Geometry: final body of the model. Coordinates: model frame, mm. A direction names the side the tool comes from. Coordinates: 2 decimals unless noted, no trailing zeros. Write each loop counter-clockwise with the first axis right and the second up, starting at its lowest first coordinate (ties: lowest second). Pieces come first, ordered by that corner, then holes. Notation, with made-up numbers: (-34, -2) - (-27, -2) arc R28 cw to (-27, 34) - close; hole circle Ø2 at (47, 83). An arc over 180 degrees is marked (long way). Put each result on its own line as item: value.
```python
from build123d import *

# Parameters (mm, degrees)
EXTRUDE_1_DEPTH    = 3
CHAMFER1_SIZE      = 110
SKETCH1_R          = 2.5
CUT_EXTRUDE1_DEPTH = 10
SKETCH2_R          = 1.6
CUT_EXTRUDE2_DEPTH = 10
CUT_EXTRUDE3_DEPTH = 10
SKETCH4_R          = 1.6
CUT_EXTRUDE4_DEPTH = 8
SKETCH5_R          = 1.5
CUT_EXTRUDE5_DEPTH = 3
SKETCH6_R          = 1.6
CUT_EXTRUDE6_DEPTH = 3
CHAMFER2_SIZE      = 10
SKETCH7_R          = 1.6
CUT_EXTRUDE7_DEPTH = 10


with BuildPart() as part:
    # 草图1 → 凸台-拉伸1 (new body)
    with BuildSketch(Plane.XY):
        Polygon((-225, 205), (-228, 205), (-228, 175), (-225, 175), (-225, 50), (-228, 50), (-228, 20), (-225, 20), (-225, -105), (-228, -105), (-228, -135), (-225, -135), (-225, -285), (225, -285), (225, -135), (228, -135), (228, -105), (225, -105), (225, 20), (228, 20), (228, 50), (225, 50), (225, 175), (228, 175), (228, 205), (225, 205), (225, 285), (-225, 285), align=None)
    extrude(amount=EXTRUDE_1_DEPTH)

    # Chamfer1
    chamfer1_edges = [part.edges().sort_by_distance(p)[0] for p in [
        (225, -285, 1.5),
        (-225, -285, 1.5),
    ]]
    chamfer(chamfer1_edges, length=CHAMFER1_SIZE)

    # Sketch1 → Cut-Extrude1 (cut)
    with BuildSketch(Plane(origin=(0, 0, 0), x_dir=(-1, 0, 0), z_dir=(0, 0, -1))):
        with Locations((102, -279.1)):
            Circle(SKETCH1_R)
        with Locations((76, -277.1)):
            Circle(SKETCH1_R)
        with Locations((50, -279.1)):
            Circle(SKETCH1_R)
        with Locations((-50, -279.1)):
            Circle(SKETCH1_R)
        with Locations((-76, -277.1)):
            Circle(SKETCH1_R)
        with Locations((-102, -279.1)):
            Circle(SKETCH1_R)
    extrude(amount=-CUT_EXTRUDE1_DEPTH, mode=Mode.SUBTRACT)

    # Sketch2 → Cut-Extrude2 (cut)
    with BuildSketch(Plane.XY.offset(3)):
        with Locations((18.5, -55)):
            Circle(SKETCH2_R)
        with Locations((-18.5, -55)):
            Circle(SKETCH2_R)
        with Locations((0, -41.5)):
            Circle(SKETCH2_R)
    extrude(amount=-CUT_EXTRUDE2_DEPTH, mode=Mode.SUBTRACT)

    # Sketch3 → Cut-Extrude3 (cut)
    with BuildSketch(Plane.XY.offset(3)):
        with BuildLine():
            Line((-12, -245), (-12, -205))
            ThreePointArc((-12, -205), (0, -193), (12, -205))
            Line((12, -205), (12, -245))
            ThreePointArc((12, -245), (0, -257), (-12, -245))
        make_face()
        with BuildLine():
            Line((-12, -120), (-12, -80))
            ThreePointArc((-12, -80), (0, -68), (12, -80))
            Line((12, -80), (12, -120))
            ThreePointArc((12, -120), (0, -132), (-12, -120))
        make_face()
    extrude(amount=-CUT_EXTRUDE3_DEPTH, mode=Mode.SUBTRACT)

    # Sketch4 → Cut-Extrude4 (cut)
    with BuildSketch(Plane.XY.offset(3)):
        with Locations((184.062077547, -179.316911543)):
            Circle(SKETCH4_R)
        with Locations((207.289508253, -167.664074122)):
            Circle(SKETCH4_R)
        with Locations((199.105034852, -143)):
            Circle(SKETCH4_R)
        with Locations((215.571067812, -30.217453576)):
            Circle(SKETCH4_R)
        with Locations((200, -20.217453576)):
            Circle(SKETCH4_R)
        with Locations((200, 7.889501876)):
            Circle(SKETCH4_R)
        with Locations((215.571067812, 17.889501876)):
            Circle(SKETCH4_R)
        with Locations((-215.571067812, 12.870402688)):
            Circle(SKETCH4_R)
        with Locations((-200, 2.870402688)):
            Circle(SKETCH4_R)
        with Locations((-200, -25.236552763)):
            Circle(SKETCH4_R)
        with Locations((-215.571067812, -35.236552763)):
            Circle(SKETCH4_R)
        with Locations((-199.105034852, -143)):
            Circle(SKETCH4_R)
        with Locations((-207.289508253, -167.664074122)):
            Circle(SKETCH4_R)
        with Locations((-184.062077547, -179.316911543)):
            Circle(SKETCH4_R)
    extrude(amount=-CUT_EXTRUDE4_DEPTH, mode=Mode.SUBTRACT)

    # Sketch5 → Cut-Extrude5 (cut)
    with BuildSketch(Plane.XY.offset(3)):
        with Locations((124.192388155, -265.908116908)):
            Circle(SKETCH5_R)
        with Locations((138.334523779, -251.765981284)):
            Circle(SKETCH5_R)
        with Locations((218, 242.361547493)):
            Circle(SKETCH5_R)
        with Locations((218, 262.361547493)):
            Circle(SKETCH5_R)
        with Locations((-218, 262.361547493)):
            Circle(SKETCH5_R)
        with Locations((-218, 242.361547493)):
            Circle(SKETCH5_R)
        with Locations((-138.334523779, -251.765981284)):
            Circle(SKETCH5_R)
        with Locations((-124.192388155, -265.908116908)):
            Circle(SKETCH5_R)
    extrude(amount=-CUT_EXTRUDE5_DEPTH, mode=Mode.SUBTRACT)

    # Sketch6 → Cut-Extrude6 (cut)
    with BuildSketch(Plane(origin=(0, 0, 0), x_dir=(-1, 0, 0), z_dir=(0, 0, -1))):
        with Locations((-28, -89.618802154)):
            Circle(SKETCH6_R)
        with Locations((28, -89.618802154)):
            Circle(SKETCH6_R)
        with Locations((28, -220.381197846)):
            Circle(SKETCH6_R)
        with Locations((-28, -220.381197846)):
            Circle(SKETCH6_R)
    extrude(amount=-CUT_EXTRUDE6_DEPTH, mode=Mode.SUBTRACT)

    # Chamfer2
    chamfer2_edges = [part.edges().sort_by_distance(p)[0] for p in [
        (-225, 285, 1.5),
        (225, 285, 1.5),
    ]]
    chamfer(chamfer2_edges, length=CHAMFER2_SIZE)

    # Sketch7 → Cut-Extrude7 (cut)
    with BuildSketch(Plane.XY.offset(3)):
        with Locations((25, -17.236552763)):
            Circle(SKETCH7_R)
        with Locations((25, -3.342800748)):
            Circle(SKETCH7_R)
        with Locations((0, 14.870402688)):
            Circle(SKETCH7_R)
        with Locations((-25, -17.236552763)):
            Circle(SKETCH7_R)
        with Locations((-25, -3.342800748)):
            Circle(SKETCH7_R)
    extrude(amount=-CUT_EXTRUDE7_DEPTH, mode=Mode.SUBTRACT)


solid = part.part
```
1. Mould query, pull axis X, two halves, no side actions, for faces 3 (the flat face through (171, -229, 1)), 4 (the flat face through (-3, 4, 3)), 5 (the cylindrical face through (0, -257, 2)). Classes: +X half, -X half, draft (parallel to the pull), parting line (faces both ways), or undercut.
Answer below:
face 3: +X half
face 4: draft
face 5: undercut
2. Ray query, probe 1 along Y at (x, z) = (-28, 0.7); probe 2 along Y at (x, z) = (0, 1.65); probe 3 along Y at (x, z) = (-200, 2.7). Return the intervals inside material, ascending. Write a range as from..to.
Answer below:
probe 1: y = -285..-221.98, -218.78..-91.22, -88.02..285
probe 2: y = -285..-257, -193..-132, -68..-43.1, -39.9..13.27, 16.47..285
probe 3: y = -200..-144.33, -141.67..-26.84, -23.64..1.27, 4.47..285
3. Pin query (flat end, axial travel): pin 1 Ø4 at (x, y) = (-124.19, -265.91) entering from -Z; pin 2 Ø0.9 at (y, z) = (-151.5, 1.5) entering from -X; pin 3 Ø0.9 at (y, z) = (257, 1.5) entering from +X; pin 4 Ø0.9 at (x, z) = (-226, 2) entering from +Y. Return the tip coordinate at first contact, or that it passes through.
Answer below:
pin 1: stops at z = 0
pin 2: stops at x = -225
pin 3: stops at x = 225
pin 4: stops at y = 205
4. Set-up query: faces 1 (the flat face through (-169, -231, 1)), 2 (the cylindrical face through (0, -193, 2)). Return all of +Z, -Z, +X, -X, +Y, -Y with unobstructed straight access to the full face (end or side cutting, diameter ignored); none if empty.
Answer below:
face 1: +Z, -Z, -X, -Y
face 2: +Z, -Z
5. Section query B-B (z = 1.9). Count the separate pieces of the cut face and the enclosed holes in it, then the cut area to 3 significant figures.
Answer below:
separate pieces: 1
enclosed holes: 42
area: 242,000 mm²
6. Section query A-A (x = -146.5). Return loops of the section in (y, z), then the cut area to 3 significant figures.
Answer below:
outline: (-253.5, 0) - (285, 0) - (285, 3) - (-253.5, 3) - close
area: 1,620 mm²
